Geometry: final body of the model. Coordinates: model frame, mm. Face numbers are marked on the shaded views. A direction names the side the tool comes from. Give positions to 0.01 mm unless a question says otherwise; leave off trailing zeros. Order: outer loops, then holes, each group sorted by start corner. A loop starts at its lowest first (then second) coordinate and runs counter-clockwise, first axis right, second up. Notation, with made-up numbers: (78, -29.75) - (124, -29.75) arc R26 cw to (124, 7.25) - close; hole circle Ø7 at (-3, 13). An arc over 180 degrees is marked (long way). Put each result on its own line as item: value. Start each with the question number.
1. Section C-C on z = -13. Return the cut outline in (x, y).
2. Set-up query: the marked faces 1 and 2. Return all of +Z, -Z, +X, -X, +Y, -Y with unobstructed straight access to the full face (end or side cutting, diameter ignored); none if empty.
3. Ray query, line 1 along X through (y, z) = (1.3, 0); line 2 along Y through (x, z) = (5.5, 0.25); line 3 along Y through (x, z) = (-2, 1). Return the intervals inside material, ascending. Write a range as from..to.
4. Section B-B on x = 7.5. Return the cut outline in (y, z).
5. First-contact query: P1, Ø1.7, axis at x = 16, z = 0, coming from the +Y side; P2, Ø5, axis at x = 0, z = 0, coming from the +Y side; P3, Ø1, axis at y = 1, z = -6.5, coming from the +X side. Flat tips, straight axial feed; report the tip coordinate or a pass-through.
6. Section A-A on y = 0.8. Count the separate pieces of the cut face and the enclosed holes in it, plus the area to 3 significant figures.
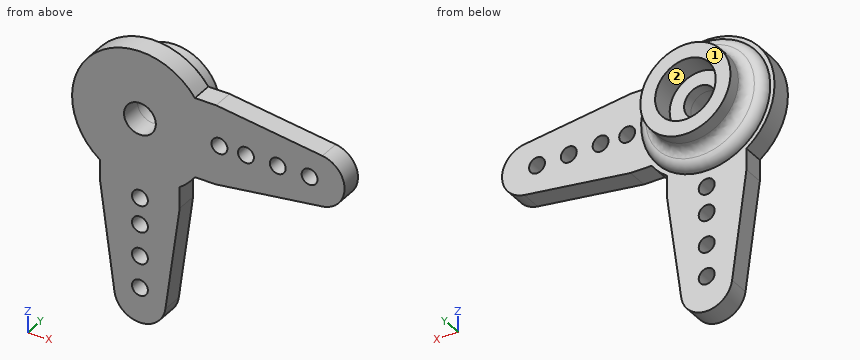
from build123d import *

# Parameters (mm, degrees)
SKETCH1_R           = 1.5
SKETCH1_R_2         = 0.75
BOSS_EXTRUDE1_DEPTH = 2
SKETCH4_R           = 4.25
SKETCH4_R_2         = 2.8575
BOSS_EXTRUDE2_DEPTH = 3.175
SKETCH5_R           = 6
BOSS_EXTRUDE3_DEPTH = 1
FILLET1_R           = 1
FILLET2_R           = 1
SKETCH7_R           = 1.5
CUT_EXTRUDE1_DEPTH  = 28.780580016


with BuildPart() as part:
    # Sketch1 → Boss-Extrude1 (new body)
    with BuildSketch(Plane(origin=(0, 0, 0), x_dir=(1, 0, 0), z_dir=(0, 1, 0))):
        with BuildLine():
            Line((-3.75, 5.186279977), (-3.75, 7.186279977))
            Line((-3.75, 7.186279977), (-2.4, 17.201793966))
            ThreePointArc((-2.4, 17.201793966), (0, 19.3), (2.4, 17.201793966))
            Line((2.4, 17.201793966), (3.75, 7.186279977))
            Line((3.75, 7.186279977), (3.75, 5.186279977))
            ThreePointArc((3.75, 5.186279977), (4.5254834, 4.5254834), (5.186279977, 3.75))
            Line((5.186279977, 3.75), (7.186279977, 3.75))
            Line((7.186279977, 3.75), (17.201793966, 2.4))
            ThreePointArc((17.201793966, 2.4), (19.3, 0), (17.201793966, -2.4))
            Line((17.201793966, -2.4), (7.186279977, -3.75))
            Line((7.186279977, -3.75), (5.186279977, -3.75))
            ThreePointArc((5.186279977, -3.75), (-4.5254834, -4.5254834), (-3.75, 5.186279977))
        make_face()
        with Locations(Location((0, 0, 0), (0, 0, 270))):
            Circle(SKETCH1_R, mode=Mode.SUBTRACT)
        with Locations(Location((0, 16, 0), (0, 0, 270))):
            Circle(SKETCH1_R_2, mode=Mode.SUBTRACT)
        with Locations(Location((0, 13, 0), (0, 0, 270))):
            Circle(SKETCH1_R_2, mode=Mode.SUBTRACT)
        with Locations(Location((0, 10, 0), (0, 0, 270))):
            Circle(SKETCH1_R_2, mode=Mode.SUBTRACT)
        with Locations(Location((0, 7.5, 0), (0, 0, 270))):
            Circle(SKETCH1_R_2, mode=Mode.SUBTRACT)
        with Locations(Location((7.5, 0, 0), (0, 0, 270))):
            Circle(SKETCH1_R_2, mode=Mode.SUBTRACT)
        with Locations(Location((10, 0, 0), (0, 0, 270))):
            Circle(SKETCH1_R_2, mode=Mode.SUBTRACT)
        with Locations(Location((13, 0, 0), (0, 0, 270))):
            Circle(SKETCH1_R_2, mode=Mode.SUBTRACT)
        with Locations(Location((16, 0, 0), (0, 0, 270))):
            Circle(SKETCH1_R_2, mode=Mode.SUBTRACT)
    extrude(amount=BOSS_EXTRUDE1_DEPTH)

    # Sketch4 → Boss-Extrude2 (add)
    with BuildSketch(Plane(origin=(0, 2, 0), x_dir=(1, 0, 0), z_dir=(0, 1, 0))):
        with Locations(Location((0, 0, 0), (0, 0, 270))):
            Circle(SKETCH4_R)
        with Locations(Location((0, 0, 0), (0, 0, 270))):
            Circle(SKETCH4_R_2, mode=Mode.SUBTRACT)
    extrude(amount=BOSS_EXTRUDE2_DEPTH)

    # Sketch5 → Boss-Extrude3 (add)
    with BuildSketch(Plane(origin=(0, 2, 0), x_dir=(1, 0, 0), z_dir=(0, 1, 0))):
        with Locations(Location((0, 0, 0), (0, 0, 270))):
            Circle(SKETCH5_R)
    extrude(amount=BOSS_EXTRUDE3_DEPTH)

    # Fillet1
    fillet1_edges = [part.edges().sort_by_distance(p)[0] for p in [
        (0, 3, -6),
    ]]
    fillet(fillet1_edges, radius=FILLET1_R - 0.0001)  # a hair under: the kernel refuses the full size

    # Fillet2
    fillet2_edges = [part.edges().sort_by_distance(p)[0] for p in [
        (0, 3, -4.25),
    ]]
    fillet(fillet2_edges, radius=FILLET2_R)

    # Sketch7 → Cut-Extrude1 (cut, through all)
    with BuildSketch(Plane.XZ):
        with Locations(Location((0, 0, 0), (0, 0, 90))):
            Circle(SKETCH7_R)
    extrude(amount=-CUT_EXTRUDE1_DEPTH, mode=Mode.SUBTRACT)


solid = part.part
Resolved:
1. outline: (-2.97, 0) - (-0.75, 0) - (-0.75, 2) - (-2.97, 2) - close; (0.75, 0) - (2.97, 0) - (2.97, 2) - (0.75, 2) - close
2. face 1: +Z, -Z, +X, -X, +Y
2. face 2: +Y
3. line 1: -6.4..-1.5, 1.5..6.75, 8.25..9.25, 10.75..12.25, 13.75..15.25, 16.75..19.3
3. line 2: 0..2.86
3. line 3: 0..3
4. outline: (0, -3.71) - (2, -3.71) - (2, -0.75) - (0, -0.75) - close; (0, 0.75) - (2, 0.75) - (2, 3.71) - (0, 3.71) - close
5. P1: y = 2
5. P2: y = 3
5. P3: x = 3.75
6. separate pieces: 1
6. enclosed holes: 9
6. area: 264 mm^2
